from build123d import *

# Parameters (mm, degrees)
SKETCH_1_W             = 34
SKETCH_1_H             = 54
SKETCH_1_R             = 2.25
EXTRUDE_1_DEPTH        = 6
SKETCH_4_W             = 8
SKETCH_4_H             = 6
EXTRUDE_2_DEPTH        = 6
SKETCH_2_W             = 22
SKETCH_2_H             = 46
CUT_EXTRUDE_1_DEPTH    = 10
FILLET_1_R             = 3
FILLET_2_R             = 2
HOLE_WIZARD_M3_1_D     = 2.5
HOLE_WIZARD_M3_1_DEPTH = 7.5
HOLE_WIZARD_M3_1_TIP   = 0.751075774
HOLE_WIZARD_M3_2_D     = 2.5
HOLE_WIZARD_M3_2_DEPTH = 101.5
HOLE_WIZARD_M3_2_TIP   = 0.751075774


with BuildPart() as part:
    # 草图1 → 凸台-拉伸1 (new body)
    with BuildSketch(Plane.XY):
        Rectangle(SKETCH_1_W, SKETCH_1_H)
        with Locations((-5, 22.75)):
            Circle(SKETCH_1_R, mode=Mode.SUBTRACT)
        with Locations(Location((5, 22.75, 0), (0, 0, 180))):
            Circle(SKETCH_1_R, mode=Mode.SUBTRACT)
    extrude(amount=EXTRUDE_1_DEPTH)

    # 草图4 → 凸台-拉伸2 (add)
    with BuildSketch(Plane.XY):
        with Locations((21, -24)):
            Rectangle(SKETCH_4_W, SKETCH_4_H)
        with Locations((-21, -24)):
            Rectangle(SKETCH_4_W, SKETCH_4_H)
    extrude(amount=EXTRUDE_2_DEPTH)

    # 草图2 → 切除-拉伸1 (cut)
    with BuildSketch(Plane.XY.offset(6)):
        with Locations((0, -4)):
            Rectangle(SKETCH_2_W, SKETCH_2_H)
    extrude(amount=-CUT_EXTRUDE_1_DEPTH, mode=Mode.SUBTRACT)

    # 圆角1
    fillet_1_edges = [part.edges().sort_by_distance(p)[0] for p in [
        (-17, 27, 3),
        (17, 27, 3),
    ]]
    fillet(fillet_1_edges, radius=FILLET_1_R)

    # 圆角2
    fillet_2_edges = [part.edges().sort_by_distance(p)[0] for p in [
        (-11, 19, 3),
        (11, 19, 3),
    ]]
    fillet(fillet_2_edges, radius=FILLET_2_R)

    # M3 螺纹孔1
    with Locations(Plane(origin=(0, -21, 0), x_dir=(1, 0, 0), z_dir=(0, 1, 0))):
        with Locations((-21, -3), (21, -3)):
            Hole(HOLE_WIZARD_M3_1_D / 2, depth=HOLE_WIZARD_M3_1_DEPTH)
            with Locations((0, 0, -(HOLE_WIZARD_M3_1_DEPTH + HOLE_WIZARD_M3_1_TIP / 2))):  # 118° drill point
                Cone(0, HOLE_WIZARD_M3_1_D / 2, HOLE_WIZARD_M3_1_TIP, mode=Mode.SUBTRACT)

    # M3 螺纹孔2
    with Locations(Plane.ZY.offset(17)):
        with Locations((3, -16)):
            Hole(HOLE_WIZARD_M3_2_D / 2, depth=HOLE_WIZARD_M3_2_DEPTH)
            with Locations((0, 0, -(HOLE_WIZARD_M3_2_DEPTH + HOLE_WIZARD_M3_2_TIP / 2))):  # 118° drill point
                Cone(0, HOLE_WIZARD_M3_2_D / 2, HOLE_WIZARD_M3_2_TIP, mode=Mode.SUBTRACT)


solid = part.part
Verification items for the finished model (mm, model axes). A direction names the side the tool comes from. Coordinates: 2 decimals unless noted, no trailing zeros. Order: outer loops, then holes, each group sorted by start corner. A loop starts at its lowest first (then second) coordinate and runs counter-clockwise, first axis right, second up. Notation, with made-up numbers: (-40, 57.25) -> (12, 57.25) arc R16 ccw to (12, 77.25) -> close; hole circle Ø5 at (-12, 85.25). An arc over 180 degrees is marked (long way). Use CSV: the item, a comma, the result in double quotes. Start each with the question number.
Q1. Section check D-D, the plane y = 14.5. Record the cut outline in (x, z).
Q2. Tool access check on faces 1 (the flat face through (20.9, -21, 1.6)), 2 (the flat face through (18, -27, 3)), 3 (the flat face through (11, -5, 3)). Record the directions out of +Z, -Z, +X, -X, +Y, -Y that give a thin tool (end or side, any length) a straight path to the whole face; none if there is none.
Q3. Section check B-B, the plane x = 5. Record the cut outline in (y, z).
Q4. Section check A-A, the plane z = 3. Give the number of separate pieces and of enclosed holes in the cut face, and give its area (3 significant figures).
Q5. Thickness scan on line 1 along X through (y, z) = (23, 1.55); line 2 along Z through (x, y) = (-21, -25); line 3 along Y through (x, z) = (-5, 3.8). Record the ranges inside material, lowest first.
Q6. Draft check along Z on faces 4 (the cylindrical face through (5, 25, 3)), 5 (the cylindrical face through (-22.155, -24.042, 3.479)), 6 (the flat face through (-11.2, 4.1, 0)), 7 (the cylindrical face through (-13.958, -14.946, 2.328)). Enter one of: +Z half, -Z half, draft (parallel to the pull), parting line (faces both ways), or undercut.
Q7. Depth check by flat-ended pin: P1, Ø1.5, axis at x = -4, z = 3.5, coming from the -Y side; P2, Ø3, axis at x = 23, z = 2.5, coming from the +Y side; P3, Ø1.8, axis at y = -12, z = 3, coming from the +X side. Enter the tip coordinate at first touch or a pass-through.
Q8. Section check C-C, the plane y = -16. Record the cut outline in (x, z), and give its area (3 significant figures).
Returned:
1,outline,"(-17, 0) -> (-11, 0) -> (-11, 6) -> (-17, 6) -> close; (11, 0) -> (17, 0) -> (17, 6) -> (11, 6) -> close"
2,face 1,"+Z, -Z, +X, +Y"
2,face 2,"+Z, -Z, +X, -X, -Y"
2,face 3,"+Z, -Z, -Y"
3,outline,"(19, 0) -> (20.5, 0) -> (20.5, 6) -> (19, 6) -> close; (25, 0) -> (27, 0) -> (27, 6) -> (25, 6) -> close"
4,separate pieces,"5"
4,enclosed holes,"2"
4,area,"826 mm^2"
5,line 1,"x = -17 to -7.24, -2.76 to 2.76, 7.24 to 17"
5,line 2,"z = 0 to 1.75, 4.25 to 6"
5,line 3,"y = 19 to 20.5, 25 to 27"
6,face 4,"draft"
6,face 5,"undercut"
6,face 6,"-Z half"
6,face 7,"undercut"
7,P1,"stops at y = 19"
7,P2,"stops at y = -21"
7,P3,"stops at x = 17"
8,outline,"(-17, 0) -> (-11, 0) -> (-11, 1.75) -> (-17, 1.75) -> close; (-17, 4.25) -> (-11, 4.25) -> (-11, 6) -> (-17, 6) -> close; (11, 0) -> (17, 0) -> (17, 1.75) -> (11, 1.75) -> close; (11, 4.25) -> (17, 4.25) -> (17, 6) -> (11, 6) -> close"
8,area,"42.0 mm^2"
